Design review of the part built by this model. Coordinates are the model's own, in mm. Give positions to 0.01 mm unless a question says otherwise; leave off trailing zeros. Loops run counter-clockwise (first coordinate to the right, second up) from the corner with the lowest first, then second, coordinate; pieces in that order, holes last. Notation, with made-up numbers: M 17,-33.75 L 31,-33.75 A17 cw 31,-1.75 Z; hole C 57,74.5 d11. An arc over 180 degrees is marked long. Answer as CSV lines item,"result".
```python
from build123d import *

# Parameters (mm, degrees)
SKETCH1_R           = 3.175
SKETCH1_R_2         = 2.999994
BOSS_EXTRUDE1_DEPTH = 6.35


with BuildPart() as part:
    # Sketch1 → Boss-Extrude1 (new body)
    with BuildSketch(Plane(origin=(0, 0, 0), x_dir=(1, 0, 0), z_dir=(0, 1, 0))):
        with BuildLine():
            Line((-254.430272712, 52.159060564), (-254.430272712, -83.730939436))
            Line((-254.430272712, -83.730939436), (-254.430272712, -90.080939436))
            Line((-254.430272712, -90.080939436), (-229.030272712, -90.080939436))
            Line((-229.030272712, -90.080939436), (-229.030272712, -83.730939436))
            Line((-229.030272712, -83.730939436), (-217.85420239, -83.730939436))
            Line((-217.85420239, -83.730939436), (-217.85420239, -80.555939436))
            Line((-217.85420239, -80.555939436), (-219.60680239, -80.555939436))
            Line((-219.60680239, -80.555939436), (-219.60680239, -78.015939436))
            Line((-219.60680239, -78.015939436), (-217.85420239, -78.015939436))
            Line((-217.85420239, -78.015939436), (-217.85420239, -76.745939436))
            Line((-217.85420239, -76.745939436), (-214.806343034, -76.745939436))
            Line((-214.806343034, -76.745939436), (-214.806343034, -78.015939436))
            Line((-214.806343034, -78.015939436), (-213.053743034, -78.015939436))
            Line((-213.053743034, -78.015939436), (-213.053743034, -80.555939436))
            Line((-213.053743034, -80.555939436), (-214.806343034, -80.555939436))
            Line((-214.806343034, -80.555939436), (-214.806343034, -83.730939436))
            Line((-214.806343034, -83.730939436), (-203.630272712, -83.730939436))
            Line((-203.630272712, -83.730939436), (-203.630272712, -90.080939436))
            Line((-203.630272712, -90.080939436), (-178.230272712, -90.080939436))
            Line((-178.230272712, -90.080939436), (-178.230272712, -83.730939436))
            Line((-178.230272712, -83.730939436), (-167.05420239, -83.730939436))
            Line((-167.05420239, -83.730939436), (-167.05420239, -80.555939436))
            Line((-167.05420239, -80.555939436), (-168.80680239, -80.555939436))
            Line((-168.80680239, -80.555939436), (-168.80680239, -78.015939436))
            Line((-168.80680239, -78.015939436), (-167.05420239, -78.015939436))
            Line((-167.05420239, -78.015939436), (-167.05420239, -76.745939436))
            Line((-167.05420239, -76.745939436), (-164.006343034, -76.745939436))
            Line((-164.006343034, -76.745939436), (-164.006343034, -78.015939436))
            Line((-164.006343034, -78.015939436), (-162.253743034, -78.015939436))
            Line((-162.253743034, -78.015939436), (-162.253743034, -80.555939436))
            Line((-162.253743034, -80.555939436), (-164.006343034, -80.555939436))
            Line((-164.006343034, -80.555939436), (-164.006343034, -83.730939436))
            Line((-164.006343034, -83.730939436), (-152.830272712, -83.730939436))
            Line((-152.830272712, -83.730939436), (-152.830272712, -90.080939436))
            Line((-152.830272712, -90.080939436), (-127.430272712, -90.080939436))
            Line((-127.430272712, -90.080939436), (-127.430272712, -83.730939436))
            Line((-127.430272712, -83.730939436), (-116.25420239, -83.730939436))
            Line((-116.25420239, -83.730939436), (-116.25420239, -80.555939436))
            Line((-116.25420239, -80.555939436), (-118.00680239, -80.555939436))
            Line((-118.00680239, -80.555939436), (-118.00680239, -78.015939436))
            Line((-118.00680239, -78.015939436), (-116.25420239, -78.015939436))
            Line((-116.25420239, -78.015939436), (-116.25420239, -76.745939436))
            Line((-116.25420239, -76.745939436), (-113.206343034, -76.745939436))
            Line((-113.206343034, -76.745939436), (-113.206343034, -78.015939436))
            Line((-113.206343034, -78.015939436), (-111.453743034, -78.015939436))
            Line((-111.453743034, -78.015939436), (-111.453743034, -80.555939436))
            Line((-111.453743034, -80.555939436), (-113.206343034, -80.555939436))
            Line((-113.206343034, -80.555939436), (-113.206343034, -83.730939436))
            Line((-113.206343034, -83.730939436), (-102.030272712, -83.730939436))
            Line((-102.030272712, -83.730939436), (-102.030272712, -90.080939436))
            Line((-102.030272712, -90.080939436), (-76.630272712, -90.080939436))
            Line((-76.630272712, -90.080939436), (-76.630272712, -83.730939436))
            Line((-76.630272712, -83.730939436), (228.169727288, -83.730939436))
            ThreePointArc((228.169727288, -83.730939436), (255.110495652, -72.571707799), (266.269727288, -45.630939436))
            Line((266.269727288, -45.630939436), (266.269727288, 14.059060564))
            ThreePointArc((266.269727288, 14.059060564), (255.110495652, 40.999828928), (228.169727288, 52.159060564))
            Line((228.169727288, 52.159060564), (-76.630272712, 52.159060564))
            Line((-76.630272712, 52.159060564), (-76.630272712, 58.509060564))
            Line((-76.630272712, 58.509060564), (-102.030272712, 58.509060564))
            Line((-102.030272712, 58.509060564), (-102.030272712, 52.159060564))
            Line((-102.030272712, 52.159060564), (-113.206343034, 52.159060564))
            Line((-113.206343034, 52.159060564), (-113.206343034, 48.984060564))
            Line((-113.206343034, 48.984060564), (-111.453743034, 48.984060564))
            Line((-111.453743034, 48.984060564), (-111.453743034, 46.444060564))
            Line((-111.453743034, 46.444060564), (-113.206343034, 46.444060564))
            Line((-113.206343034, 46.444060564), (-113.206343034, 45.174060564))
            Line((-113.206343034, 45.174060564), (-116.25420239, 45.174060564))
            Line((-116.25420239, 45.174060564), (-116.25420239, 46.444060564))
            Line((-116.25420239, 46.444060564), (-118.00680239, 46.444060564))
            Line((-118.00680239, 46.444060564), (-118.00680239, 48.984060564))
            Line((-118.00680239, 48.984060564), (-116.25420239, 48.984060564))
            Line((-116.25420239, 48.984060564), (-116.25420239, 52.159060564))
            Line((-116.25420239, 52.159060564), (-127.430272712, 52.159060564))
            Line((-127.430272712, 52.159060564), (-127.430272712, 58.509060564))
            Line((-127.430272712, 58.509060564), (-152.830272712, 58.509060564))
            Line((-152.830272712, 58.509060564), (-152.830272712, 52.159060564))
            Line((-152.830272712, 52.159060564), (-164.006343034, 52.159060564))
            Line((-164.006343034, 52.159060564), (-164.006343034, 48.984060564))
            Line((-164.006343034, 48.984060564), (-162.253743034, 48.984060564))
            Line((-162.253743034, 48.984060564), (-162.253743034, 46.444060564))
            Line((-162.253743034, 46.444060564), (-164.006343034, 46.444060564))
            Line((-164.006343034, 46.444060564), (-164.006343034, 45.174060564))
            Line((-164.006343034, 45.174060564), (-167.05420239, 45.174060564))
            Line((-167.05420239, 45.174060564), (-167.05420239, 46.444060564))
            Line((-167.05420239, 46.444060564), (-168.80680239, 46.444060564))
            Line((-168.80680239, 46.444060564), (-168.80680239, 48.984060564))
            Line((-168.80680239, 48.984060564), (-167.05420239, 48.984060564))
            Line((-167.05420239, 48.984060564), (-167.05420239, 52.159060564))
            Line((-167.05420239, 52.159060564), (-178.230272712, 52.159060564))
            Line((-178.230272712, 52.159060564), (-178.230272712, 58.509060564))
            Line((-178.230272712, 58.509060564), (-203.630272712, 58.509060564))
            Line((-203.630272712, 58.509060564), (-203.630272712, 52.159060564))
            Line((-203.630272712, 52.159060564), (-214.806343034, 52.159060564))
            Line((-214.806343034, 52.159060564), (-214.806343034, 48.984060564))
            Line((-214.806343034, 48.984060564), (-213.053743034, 48.984060564))
            Line((-213.053743034, 48.984060564), (-213.053743034, 46.444060564))
            Line((-213.053743034, 46.444060564), (-214.806343034, 46.444060564))
            Line((-214.806343034, 46.444060564), (-214.806343034, 45.174060564))
            Line((-214.806343034, 45.174060564), (-217.85420239, 45.174060564))
            Line((-217.85420239, 45.174060564), (-217.85420239, 46.444060564))
            Line((-217.85420239, 46.444060564), (-219.60680239, 46.444060564))
            Line((-219.60680239, 46.444060564), (-219.60680239, 48.984060564))
            Line((-219.60680239, 48.984060564), (-217.85420239, 48.984060564))
            Line((-217.85420239, 48.984060564), (-217.85420239, 52.159060564))
            Line((-217.85420239, 52.159060564), (-229.030272712, 52.159060564))
            Line((-229.030272712, 52.159060564), (-229.030272712, 58.509060564))
            Line((-229.030272712, 58.509060564), (-254.430272712, 58.509060564))
            Line((-254.430272712, 58.509060564), (-254.430272712, 52.159060564))
        make_face()
        with Locations(Location((240.869727288, 8.026560564, 0), (0, 0, 270))):
            Circle(SKETCH1_R, mode=Mode.SUBTRACT)
        with Locations(Location((240.869727288, -39.598439436, 0), (0, 0, 270))):
            Circle(SKETCH1_R, mode=Mode.SUBTRACT)
        with Locations(Location((-51.230272712, -40.550939436, 0), (0, 0, 270))):
            Circle(SKETCH1_R, mode=Mode.SUBTRACT)
        with Locations(Location((-51.230272712, 8.979060564, 0), (0, 0, 270))):
            Circle(SKETCH1_R, mode=Mode.SUBTRACT)
        with Locations(Location((-247.430286712, 8.714138564, 0), (0, 0, 270))):
            Circle(SKETCH1_R_2, mode=Mode.SUBTRACT)
        with Locations(Location((-247.430286712, -40.286017436, 0), (0, 0, 270))):
            Circle(SKETCH1_R_2, mode=Mode.SUBTRACT)
        with Locations(Location((-81.430364712, 8.714138564, 0), (0, 0, 270))):
            Circle(SKETCH1_R_2, mode=Mode.SUBTRACT)
        with Locations(Location((-81.430364712, -40.286017436, 0), (0, 0, 270))):
            Circle(SKETCH1_R_2, mode=Mode.SUBTRACT)
        Polygon((-76.630272712, -15.785939436), (-76.630272712, -3.085939436), (-82.959141148, -3.085939436), (-82.959141148, -28.485939436), (-76.630272712, -28.485939436), align=None, mode=Mode.SUBTRACT)
    extrude(amount=BOSS_EXTRUDE1_DEPTH)


solid = part.part
```
1. We need section B-B, the plane y = 4.75. Count the separate pieces of the cut face and the enclosed holes in it, plus the area to 3 significant figures.
Answer block:
separate pieces,"1"
enclosed holes,"9"
area,"70,800 mm²"
2. To check wall thickness, follow L1, parallel to Z at x = -83, y = 6; L2, parallel to Z at x = 49.5, y = 2; L3, parallel to X at y = 1.25, z = 20. State the ranges of each line that lie inside material, in increasing order. Write a range as [from, to].
Answer block:
L1,"[-58.51, -11.27], [-6.16, 37.73], [42.84, 90.08]"
L2,"[-52.16, 83.73]"
L3,"[-254.43, -82.96], [-76.63, 266.27]"
3. We need section A-A, the plane x = 162. Write out the cut boundary in (y, z).
Answer block:
outline,"M 0,-52.16 L 6.35,-52.16 L 6.35,83.73 L 0,83.73 Z"
4. For P1, Ø0.9, axis at x = -117.5, y = 4.5, coming from the -Z side; P2, Ø0.9, axis at x = -165.5, y = 3, coming from the -Z side; P3, Ø3, axis at y = 2.5, z = 87.5, coming from the +X side, all flat-tipped, find the tip position at first contact; note any pin that passes through.
Answer block:
P1,"z = -52.16"
P2,"z = -45.17"
P3,"x = -76.63"
